Check sheet for the modelled part. Datum: model origin and axes. Units: mm. A direction names the side the tool comes from. Round coordinates to 2 decimals unless told otherwise and drop trailing zeros. Order: outer loops, then holes, each group sorted by start corner. A loop starts at its lowest first (then second) coordinate and runs counter-clockwise, first axis right, second up.
from build123d import *

# Parameters (mm, degrees)
BOSS_EXTRUDE1_DEPTH = 8
SKETCH2_R           = 1.55
CUT_EXTRUDE1_DEPTH  = 18.549928775
FILLET1_R           = 3
FILLET2_R           = 3
FILLET3_R           = 1
FILLET4_R           = 0.5


with BuildPart() as part:
    # Sketch1 → Boss-Extrude1 (new body)
    with BuildSketch(Plane.XY):
        with BuildLine():
            Line((-5, -1.5), (-5, 0))
            Line((-5, 0), (-5, 1.5))
            ThreePointArc((-5, 1.5), (0, 6.5), (5, 1.5))
            Line((5, 1.5), (5, 0))
            Line((5, 0), (5, -1.5))
            Line((5, -1.5), (12, -1.5))
            Line((12, -1.5), (12, 1.5))
            Line((12, 1.5), (7, 1.5))
            ThreePointArc((7, 1.5), (0, 8.5), (-7, 1.5))
            Line((-7, 1.5), (-12, 1.5))
            Line((-12, 1.5), (-12, -1.5))
            Line((-12, -1.5), (-5, -1.5))
        make_face()
    extrude(amount=BOSS_EXTRUDE1_DEPTH)

    # Sketch2 → Cut-Extrude1 (cut, through all)
    with BuildSketch(Plane.XZ.offset(1.5)):
        with Locations(Location((-8.5, 4, 0), (0, 0, 270))):
            Circle(SKETCH2_R)
        with Locations(Location((8.5, 4, 0), (0, 0, 270))):
            Circle(SKETCH2_R)
    extrude(amount=-CUT_EXTRUDE1_DEPTH, mode=Mode.SUBTRACT)

    # Fillet1
    # the kernel refuses this fillet: 3 mm, written as the material it adds along each edge
    with BuildSketch(Plane(origin=(-7, 1.5, -1.957967552), x_dir=(-1, 0, 0), z_dir=(0, 0, 1))) as fillet1_piece_1_section:
        with BuildLine():
            CenterArc((2.539392014, -3), FILLET1_R, 90, 72.542396876)
            ThreePointArc((-0.32242559, -2.1), (-0.081075919, -1.062303895), (0, 0))
            Line((0, 0), (2.539392014, 0))
        make_face()
    fillet1_piece_1 = extrude(amount=9.957967552, mode=Mode.PRIVATE)
    fillet1_piece_1 = split(fillet1_piece_1, bisect_by=Plane(origin=(-8.907059095, 1.548017233, 0), z_dir=(0, 0, 1)), keep=Keep.TOP, mode=Mode.PRIVATE)
    fillet1_piece_1 = fillet1_piece_1 - Plane(origin=(-8.5, 1.548017233, 4), x_dir=(0, 0, -1), z_dir=(0, -1, 0)) * Cylinder(1.55, 31, mode=Mode.PRIVATE)
    add(fillet1_piece_1)
    with BuildSketch(Plane(origin=(-7, 1.5, 0), x_dir=(-1, 0, 0), z_dir=(0, 0, 1))) as fillet1_piece_2_section:
        with BuildLine():
            CenterArc((2.539392014, -3), FILLET1_R, 90, 72.542396876)
            ThreePointArc((-0.32242559, -2.1), (-0.081075919, -1.062303895), (0, 0))
            Line((0, 0), (2.539392014, 0))
        make_face()
    fillet1_piece_2 = extrude(amount=9.957967552, mode=Mode.PRIVATE)
    fillet1_piece_2 = split(fillet1_piece_2, bisect_by=Plane(origin=(-8.907059095, 1.548017233, 8), z_dir=(0, 0, -1)), keep=Keep.TOP, mode=Mode.PRIVATE)
    fillet1_piece_2 = fillet1_piece_2 - Plane(origin=(-8.5, 1.548017233, 4), x_dir=(0, 0, -1), z_dir=(0, -1, 0)) * Cylinder(1.55, 31, mode=Mode.PRIVATE)
    add(fillet1_piece_2)
    with BuildSketch(Plane(origin=(7, 1.5, -1.957967552), x_dir=(-0.15175769928250127, 0.9884177258166114, 0), z_dir=(0, 0, 1))) as fillet1_piece_3_section:
        with BuildLine():
            CenterArc((2.579880888, -2.965253177), FILLET1_R, 98.728801562, 72.542396876)
            Line((-0.38537229, -2.50998008), (0, 0))
            ThreePointArc((0, 0), (1.062303895, -0.081075919), (2.12460779, 0))
        make_face()
    fillet1_piece_3 = extrude(amount=9.957967552, mode=Mode.PRIVATE)
    fillet1_piece_3 = split(fillet1_piece_3, bisect_by=Plane(origin=(6.913079809, 3.011198011, 0), z_dir=(0, 0, 1)), keep=Keep.TOP, mode=Mode.PRIVATE)
    fillet1_piece_3 = fillet1_piece_3 - Plane(origin=(8.5, 3.011198011, 4), x_dir=(0, 0, -1), z_dir=(0, -1, 0)) * Cylinder(1.55, 30, mode=Mode.PRIVATE)
    add(fillet1_piece_3)
    with BuildSketch(Plane(origin=(7, 1.5, 0), x_dir=(-0.15175769928250127, 0.9884177258166114, 0), z_dir=(0, 0, 1))) as fillet1_piece_4_section:
        with BuildLine():
            CenterArc((2.579880888, -2.965253177), FILLET1_R, 98.728801562, 72.542396876)
            Line((-0.38537229, -2.50998008), (0, 0))
            ThreePointArc((0, 0), (1.062303895, -0.081075919), (2.12460779, 0))
        make_face()
    fillet1_piece_4 = extrude(amount=9.957967552, mode=Mode.PRIVATE)
    fillet1_piece_4 = split(fillet1_piece_4, bisect_by=Plane(origin=(6.913079809, 3.011198011, 8), z_dir=(0, 0, -1)), keep=Keep.TOP, mode=Mode.PRIVATE)
    fillet1_piece_4 = fillet1_piece_4 - Plane(origin=(8.5, 3.011198011, 4), x_dir=(0, 0, -1), z_dir=(0, -1, 0)) * Cylinder(1.55, 30, mode=Mode.PRIVATE)
    add(fillet1_piece_4)

    # Fillet2
    # the kernel refuses this fillet: 3 mm, written as the material it takes off along each edge
    with BuildSketch(Plane(origin=(-12, 9, 0), x_dir=(1, 0, 0), z_dir=(0, -1, 0)), Plane(origin=(12, -9, 0), x_dir=(-1, 0, 0), z_dir=(0, 1, 0))) as fillet2_piece_1:
        with BuildLine():
            CenterArc((FILLET2_R, FILLET2_R), FILLET2_R, 180, 90)
            Line((0, FILLET2_R), (0, 0))
            Line((0, 0), (FILLET2_R, 0))
        make_face()
    extrude(amount=18, mode=Mode.SUBTRACT)
    with BuildSketch(Plane(origin=(-12, 9, 8), x_dir=(1, 0, 0), z_dir=(0, -1, 0)), Plane(origin=(12, -9, 8), x_dir=(-1, 0, 0), z_dir=(0, 1, 0))) as fillet2_piece_2:
        with BuildLine():
            CenterArc((FILLET2_R, -FILLET2_R), FILLET2_R, 90, 90)
            Line((0, -FILLET2_R), (0, 0))
            Line((0, 0), (FILLET2_R, 0))
        make_face()
    extrude(amount=18, mode=Mode.SUBTRACT)

    # Fillet3
    fillet3_edges = [part.edges().sort_by_distance(p)[0] for p in [
        (5, 0, 0),
        (0, 6.5, 0),
        (-5, 0, 0),
        (-5, 0, 8),
        (0, 6.5, 8),
        (5, 0, 8),
    ]]
    fillet(fillet3_edges, radius=FILLET3_R)

    # Fillet4
    fillet4_edges = [part.edges().sort_by_distance(p)[0] for p in [
        (0, 8.5, 8),
        (0, 8.5, 0),
        (-7.553486472, 2.251405066, 8),
        (7.553486472, 2.251405066, 0),
        (7.553486472, 2.251405066, 8),
        (-12, 1.5, 4),
        (-11.304145833, 1.5, 1.078825365),
        (-11.304145833, 1.5, 6.921174635),
        (-7.553486472, 2.251405066, 0),
        (-9.269696007, 1.512147249, 0.012147249),
        (-9.269696007, 1.512147249, 7.987852751),
        (12, 1.5, 4),
        (9.269696008, 1.512147249, 0.012147249),
        (9.269696008, 1.512147249, 7.987852751),
        (11.304145833, 1.5, 1.078825365),
        (11.304145833, 1.5, 6.921174635),
    ]]
    fillet(fillet4_edges, radius=FILLET4_R)


solid = part.part
1) Gauge pin test, flat ends, axial feed: pin 1 (4 mm diameter, centred on y = 2.5, z = 6, fed in from -X); pin 2 (1.6 mm diameter, centred on x = 10.5, z = 4, fed in from +Y); pin 3 (2 mm diameter, centred on y = 1.5, z = 1, fed in from +X). Record the tip position at first contact, or that the pin passes through.
2) Draft check along X on faces 1 (the face through (-6.94, 3, 3.17)), 2 (the face through (11.1, -0.25, 7.14)), 3 (the face through (-0.1, 6.5, 4)). Enter one of: pulls with the +X half, pulls with the -X half, needs draft (parallel to the pull), parting line crosses it, or undercut.
3) Sectioned sample at A-A on x = 0. Record the cut outline in (y, z).
4) Set-up check for faces 4 (the face through (11, 1.5, 4)), 5 (the face through (-5.301, 0.021, 0.285)), 6 (the face through (5.301, -0.021, 7.715)), 7 (the face through (5, 0, 4)), 8 (the face through (11.14, -0.25, 0.9)): record each of +Z, -Z, +X, -X, +Y, -Y from which the full face is reachable in a straight line by a thin tool's end or side.
5) Sectioned sample at B-B on z = 4.75. Record the cut outline in (x, y).
6) Scan lines: line 1 (X direction, y = 0.35, z = 4); line 2 (Z direction, x = 8.5, y = 0.9); line 3 (X direction, y = 3.5, z = 2). Record each from-to range of solid material in increasing order.
Values found:
1. pin 1: stops at x = -12
1. pin 2: stops at y = 1.5
1. pin 3: stops at x = 11.79
2. face 1: pulls with the -X half
2. face 2: pulls with the +X half
2. face 3: undercut
3. outline: (6.5, 1) arc R1 ccw to (7.5, 0) - (8, 0) arc R0.5 ccw to (8.5, 0.5) - (8.5, 7.5) arc R0.5 ccw to (8, 8) - (7.5, 8) arc R1 ccw to (6.5, 7) - close
4. face 4: +Z, -Z, +X, +Y
4. face 5: -Z, -Y
4. face 6: +Z, -Y
4. face 7: +Z, -Z, -Y
4. face 8: -Z, +X, +Y, -Y
5. outline: (-12, -1.5) - (-9.86, -1.5) - (-9.86, 1.5) - (-11.5, 1.5) arc R0.5 ccw to (-12, 1) - close; (-7.14, -1.5) - (-5, -1.5) - (-5, 1.5) arc R5 cw to (5, 1.5) - (5, -1.5) - (7.14, -1.5) - (7.14, 2.69) arc R3 cw to (6.68, 3.6) arc R7 ccw to (-6.68, 3.6) arc R3 cw to (-7.14, 2.69) - close; (9.86, -1.5) - (12, -1.5) - (12, 1) arc R0.5 ccw to (11.5, 1.5) - (9.86, 1.5) - close
6. line 1: x = -12 to -10.05, -6.95 to -5, 5 to 6.95, 10.05 to 12
6. line 2: z = 0 to 2.45, 5.55 to 8
6. line 3: x = -6.71 to -4.58, 4.58 to 6.71
